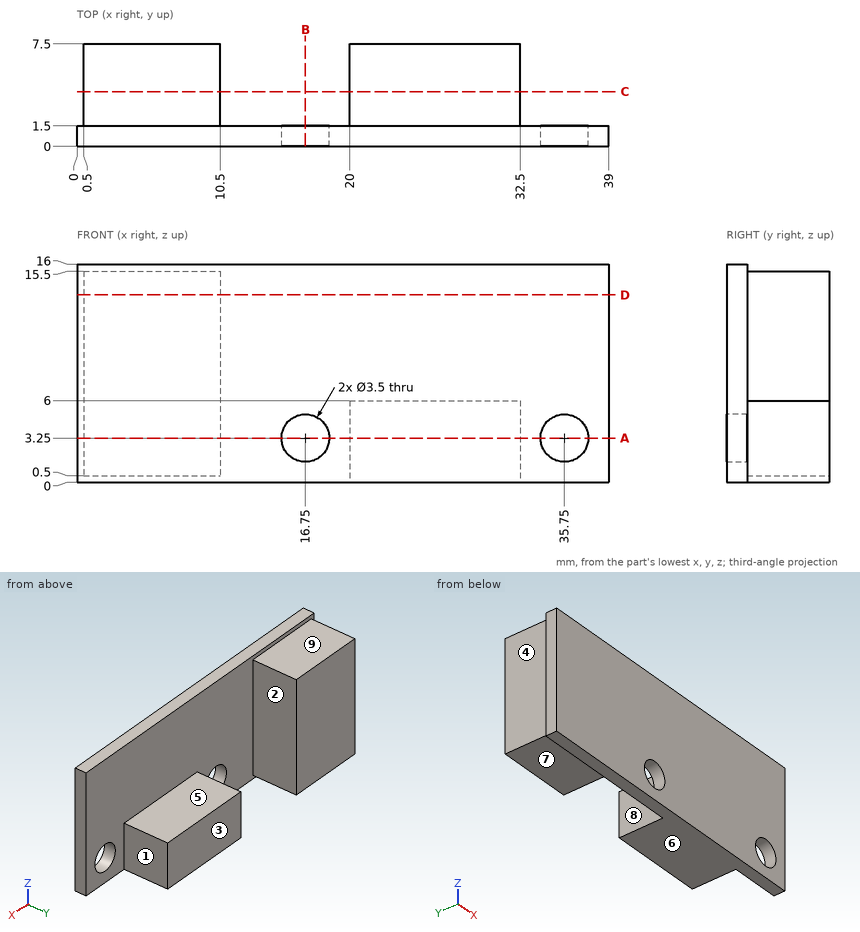
For this review, use the dimensioned drawing (mm, ordinates from the lowest corner) and the shaded views. A direction names the side the tool comes from. Give positions to 0.01 mm unless a question says otherwise; leave off trailing zeros. Order: outer loops, then holes, each group sorted by start corner. A loop starts at its lowest first (then second) coordinate and runs counter-clockwise, first axis right, second up. Notation, with made-up numbers: (-39, 17) -> (-8, 17) arc R9 cw to (-8, 33) -> close; hole circle Ø10 at (36.25, 17.5). An arc over 180 degrees is marked (long way). Write item = value, one per line. Start each with the question number.
(1) Take a section at B-B (x = 16.75). Write out the cut boundary in (y, z), plus the area to 4 significant figures.
(2) Tool access review of the marked faces 5, 6, 7, 8 and 9: name each direction out of +Z, -Z, +X, -X, +Y, -Y from which nothing blocks a thin tool from reaching the whole face with its end or side.
(3) Draft analysis for pull direction X (two halves, no side actions). For the marked faces 1, 2, 3 and 4, state which applies: +X half, -X half, draft (parallel to the pull), parting line (faces both ways), or undercut.
(4) For pin 1 Ø1.8 at (y, z) = (4, 4) entering from -X; pin 2 Ø1.5 at (y, z) = (1, 9.5) entering from -X; pin 3 Ø1.8 at (y, z) = (4.5, 11) entering from +X; pin 4 Ø4 at (x, y) = (24.5, 5) entering from +Z, all flat-tipped, find the tip position at first contact; note any pin that passes through.
(5) Take a section at D-D (z = 13.75). Write out the cut boundary in (x, y), plus the area to 4 significant figures.
(6) For L1, parallel to X at y = 0.4, z = 3.25; L2, parallel to X at y = 3, z = 5.25; L3, parallel to Y at x = 26, z = 6.5, list the stretches that pass through material, from the lowest coordinate up. Write a range as from..to.
(7) Take a section at A-A (z = 3.25). Write out the cut boundary in (x, y), plus the area to 3 significant figures.
(8) Take a section at C-C (y = 4). Write out the cut boundary in (x, z).
Returned:
q1.outline = (0, 0) -> (1.5, 0) -> (1.5, 1.5) -> (0, 1.5) -> close; (0, 5) -> (1.5, 5) -> (1.5, 16) -> (0, 16) -> close
q1.area = 18.75 mm²
q2.face_5 = +Z, +X, +Y
q2.face_6 = -Z, +X, -X, +Y, -Y
q2.face_7 = -Z, -X, +Y
q2.face_8 = +Z, -Z, +Y
q2.face_9 = +Z, +X, -X, +Y
q3.face_1 = +X half
q3.face_2 = undercut
q3.face_3 = draft
q3.face_4 = -X half
q4.pin_1 = 0.5
q4.pin_2 = 0
q4.pin_3 = 10.5
q4.pin_4 = 6
q5.outline = (0, 0) -> (39, 0) -> (39, 1.5) -> (10.5, 1.5) -> (10.5, 7.5) -> (0.5, 7.5) -> (0.5, 1.5) -> (0, 1.5) -> close
q5.area = 118.5 mm²
q6.L1 = 0..15, 18.5..34, 37.5..39
q6.L2 = 0.5..10.5, 20..32.5
q6.L3 = 0..1.5
q7.outline = (0, 0) -> (15, 0) -> (15, 1.5) -> (10.5, 1.5) -> (10.5, 7.5) -> (0.5, 7.5) -> (0.5, 1.5) -> (0, 1.5) -> close; (18.5, 0) -> (34, 0) -> (34, 1.5) -> (32.5, 1.5) -> (32.5, 7.5) -> (20, 7.5) -> (20, 1.5) -> (18.5, 1.5) -> close; (37.5, 0) -> (39, 0) -> (39, 1.5) -> (37.5, 1.5) -> close
q7.area = 183 mm²
q8.outline = (0.5, 0.5) -> (10.5, 0.5) -> (10.5, 15.5) -> (0.5, 15.5) -> close; (20, 0) -> (32.5, 0) -> (32.5, 6) -> (20, 6) -> close
